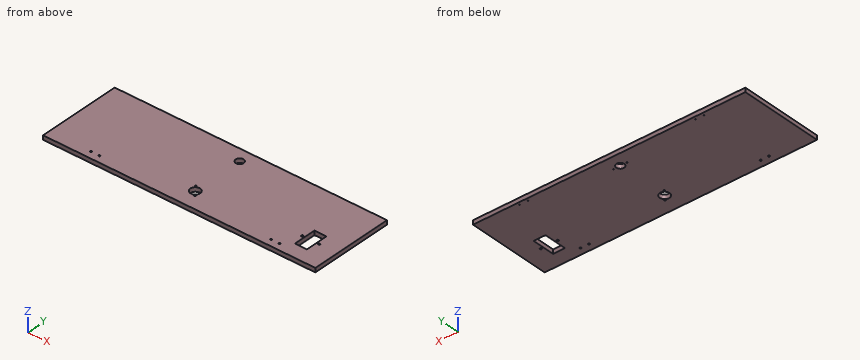
```python
from build123d import *

# Parameters (mm, degrees)
ESQUISSE1_W             = 650
ESQUISSE1_H             = 200
BOSS_EXTRU_1_DEPTH      = 10
ESQUISSE2_R             = 2
ENL_V_MAT_EXTRU_1_DEPTH = 10
ESQUISSE3_R             = 1.6
ESQUISSE3_R_2           = 11.75
ESQUISSE3_W             = 28.5
ESQUISSE3_H             = 54.3
ESQUISSE3_R_3           = 2.25
ENL_V_MAT_EXTRU_2_DEPTH = 10
ESQUISSE4_R             = 9.5
ENL_V_MAT_EXTRU_3_DEPTH = 10
ESQUISSE5_R             = 1
ENL_V_MAT_EXTRU_4_DEPTH = 2


with BuildPart() as part:
    # Esquisse1 → Boss.-Extru.1 (new body)
    with BuildSketch(Plane.XY):
        with Locations((325, 100)):
            Rectangle(ESQUISSE1_W, ESQUISSE1_H)
    extrude(amount=BOSS_EXTRU_1_DEPTH)

    # Esquisse2 → Enlèv. mat.-Extru.1 (cut)
    with BuildSketch(Plane.XY.offset(10)):
        with Locations((100, 17)):
            Circle(ESQUISSE2_R)
        with Locations((120, 17)):
            Circle(ESQUISSE2_R)
        with Locations((530, 17)):
            Circle(ESQUISSE2_R)
        with Locations((550, 17)):
            Circle(ESQUISSE2_R)
    extrude(amount=-ENL_V_MAT_EXTRU_1_DEPTH, mode=Mode.SUBTRACT)

    # Esquisse3 → Enlèv. mat.-Extru.2 (cut)
    with BuildSketch(Plane.XY.offset(10)):
        with Locations((315.499614794, 56.999404399)):
            Circle(ESQUISSE3_R)
        with Locations((325, 45)):
            Circle(ESQUISSE3_R_2)
        with Locations((334.500385206, 33.000595601)):
            Circle(ESQUISSE3_R)
        with Locations((585.75, 62.15)):
            Rectangle(ESQUISSE3_W, ESQUISSE3_H)
        with Locations((565.75, 62.15)):
            Circle(ESQUISSE3_R_3)
        with Locations((605.75, 62.15)):
            Circle(ESQUISSE3_R_3)
    extrude(amount=-ENL_V_MAT_EXTRU_2_DEPTH, mode=Mode.SUBTRACT)

    # Esquisse4 → Enlèv. mat.-Extru.3 (cut)
    with BuildSketch(Plane.XY.offset(10)):
        with Locations((325, 169)):
            Circle(ESQUISSE4_R)
    extrude(amount=-ENL_V_MAT_EXTRU_3_DEPTH, mode=Mode.SUBTRACT)

    # Esquisse5 → Enlèv. mat.-Extru.4 (cut)
    with BuildSketch(Plane.XY):
        with Locations((341, 169)):
            Circle(ESQUISSE5_R)
        with Locations((309, 169)):
            Circle(ESQUISSE5_R)
        with Locations((125, 193)):
            Circle(ESQUISSE5_R)
        with Locations((105, 193)):
            Circle(ESQUISSE5_R)
        with Locations((545, 193)):
            Circle(ESQUISSE5_R)
        with Locations((525, 193)):
            Circle(ESQUISSE5_R)
    extrude(amount=ENL_V_MAT_EXTRU_4_DEPTH, mode=Mode.SUBTRACT)


solid = part.part
```
Work out the finished part from the listing and answer in its coordinate system (mm). Give positions to 0.01 mm unless a question says otherwise; leave off trailing zeros. Order: outer loops, then holes, each group sorted by start corner. A loop starts at its lowest first (then second) coordinate and runs counter-clockwise, first axis right, second up. Notation, with made-up numbers: M 58.25,29.5 L 64.25,29.5 A14 cw 64.25,43.5 Z; hole C 3,82.25 d11. An arc over 180 degrees is marked long. Return JSON: item names as keys, results as strings.
1) Section B-B, the plane z = 5 is taken. Give the number of separate pieces and of enclosed holes in the cut face, plus the area to 3 significant figures.
Resolved:
{"separate pieces": "1", "enclosed holes": "11", "area": "128,000 mm^2"}
2) Straight lines are drawn through the part: line 1 along X through (y, z) = (193, 1.15); line 2 along Y through (x, z) = (341, 1.1); line 3 along Y through (x, z) = (595, 5.5). For each, find the intervals that lie inside material, in ascending order. Write a range as [from, to].
Resolved:
{"line 1": "[0, 104], [106, 124], [126, 524], [526, 544], [546, 650]", "line 2": "[0, 168], [170, 200]", "line 3": "[0, 35], [89.3, 200]"}
3) Section A-A, the plane y = 45 is taken. Write down the section's boundary in (x, z), plus the area to 3 significant figures.
Resolved:
{"outline": "M 0,0 L 313.25,0 L 313.25,10 L 0,10 Z; M 336.75,0 L 571.5,0 L 571.5,10 L 336.75,10 Z; M 600,0 L 650,0 L 650,10 L 600,10 Z", "area": "5,980 mm^2"}
4) Each of these flat-tipped pins is pushed along its axis until it touches: pin 1 (1 mm diameter, centred on x = 124, z = 8, fed in from -Y); pin 2 (3 mm diameter, centred on x = 550, y = 17, fed in from +Z); pin 3 (0.6 mm diameter, centred on x = 125, y = 193.5, fed in from -Z). Where does it stop, or does it pass through?
Resolved:
{"pin 1": "y = 0", "pin 2": "through", "pin 3": "z = 2"}
